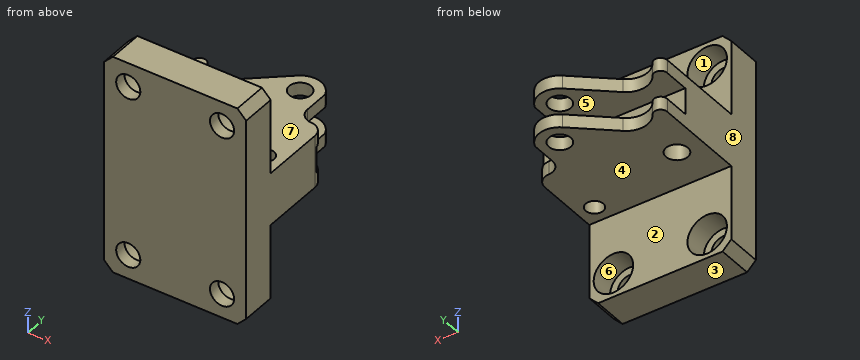
```python
from build123d import *

# Parameters (mm, degrees)
EXTRUDE_1_DEPTH              = 35
SKETCH_2_W                   = 82.468710257
SKETCH_2_H                   = 88.660900106
CUT_EXTRUDE_1_DEPTH          = 40
SKETCH_10_R                  = 2.5
CUT_EXTRUDE_6_DEPTH          = 48.259263975
SKETCH_11_R                  = 2.5
CUT_EXTRUDE_7_DEPTH          = 48.259263975
SKETCH_13_R                  = 2
CUT_EXTRUDE_8_DEPTH          = 48.259263975
FILLET_1_R                   = 3
SKETCH_14_W                  = 32.391015019
SKETCH_14_H                  = 50
EXTRUDE_2_DEPTH              = 8
CHAMFER_1_SIZE               = 2
HOLE_WIZARD_M5_1_D           = 5.5
HOLE_WIZARD_M5_1_CBORE_D     = 9
HOLE_WIZARD_M5_1_CBORE_DEPTH = 5.3


with BuildPart() as part:
    # 草圖1 → 填料-伸長1 (new body)
    with BuildSketch(Plane(origin=(0, 0, 0), x_dir=(0, 0, -1), z_dir=(1, 0, 0))):
        Polygon((-13.9, 3), (-25.9, 3), (-25.9, 38), (-22.9, 38), (-22.9, 18), (-16.9, 18), (-16.9, 38), (-13.9, 38), align=None)
    extrude(amount=-EXTRUDE_1_DEPTH)

    # 草圖2 → 除料-伸長1 (cut)
    with BuildSketch(Plane.XY.offset(13.9)):
        with Locations((-13.573394444, 11.892084287)):
            Rectangle(SKETCH_2_W, SKETCH_2_H)
        with BuildLine():
            Line((-32.391015019, 23.817806702), (-32.391015019, 3))
            Line((-32.391015019, 3), (0, 3))
            Line((0, 3), (0, 20.4))
            Line((0, 20.4), (-2.9, 20.4))
            ThreePointArc((-2.9, 20.4), (-5.021320344, 21.278679656), (-5.9, 23.4))
            Line((-5.9, 23.4), (-5.9, 29.121329309))
            ThreePointArc((-5.9, 29.121329309), (-9.201633351, 32.099001439), (-13.531412968, 31.088891261))
            Line((-13.531412968, 31.088891261), (-22.178800852, 23.645419036))
            ThreePointArc((-22.178800852, 23.645419036), (-26.149318252, 22.485359315), (-29.634828865, 24.712905667))
            ThreePointArc((-29.634828865, 24.712905667), (-31.356390105, 25.322962362), (-32.391015019, 23.817806702))
        make_face(mode=Mode.SUBTRACT)
    extrude(amount=CUT_EXTRUDE_1_DEPTH, mode=Mode.SUBTRACT)

    # 草圖10 → 除料-伸長6 (cut, through all)
    with BuildSketch(Plane.XY.offset(25.9)):
        with Locations((-10.44068936, 27.5)):
            Circle(SKETCH_10_R)
    extrude(amount=-CUT_EXTRUDE_6_DEPTH, mode=Mode.SUBTRACT)

    # 草圖11 → 除料-伸長7 (cut, through all)
    with BuildSketch(Plane.XY.offset(25.9)):
        with Locations((-26.54068936, 12.35)):
            Circle(SKETCH_11_R)
    extrude(amount=-CUT_EXTRUDE_7_DEPTH, mode=Mode.SUBTRACT)

    # 草圖13 → 除料-伸長8 (cut, through all)
    with BuildSketch(Plane.XY.offset(25.9)):
        with Locations((-4, 7)):
            Circle(SKETCH_13_R)
    extrude(amount=-CUT_EXTRUDE_8_DEPTH, mode=Mode.SUBTRACT)

    # 圓角1
    # the kernel refuses this fillet: 3 mm, written as the material it takes off along each edge
    with BuildSketch(Plane(origin=(0, 20.4, 15.402083478), x_dir=(0, -1, 0), z_dir=(0, 0, 1)), Plane(origin=(0, 20.4, 6.402083478), x_dir=(0, -1, 0), z_dir=(0, 0, 1))) as fillet_1_piece_1:
        with BuildLine():
            CenterArc((2.999166609, -3), FILLET_1_R, 90, 89.045026126)
            Line((-0.000416696, -2.95), (-0.300375026, -2.945))
            ThreePointArc((-0.300375026, -2.945), (-0.3, -2.9), (-0.3, 0))
            Line((-0.3, 0), (0, 0.3))
            Line((0, 0.3), (2.999166609, 0.3))
            Line((2.999166609, 0.3), (2.999166609, 0))
        make_face()
    extrude(amount=17.995833044, mode=Mode.SUBTRACT)

    # 草圖14 → 填料-伸長2 (add)
    with BuildSketch(Plane.XZ.offset(-3)):
        with Locations((-16.19550751, 19.9)):
            Rectangle(SKETCH_14_W, SKETCH_14_H)
    extrude(amount=EXTRUDE_2_DEPTH)

    # 導角1
    chamfer_1_edges = [part.edges().sort_by_distance(p)[0] for p in [
        (-32.391015019, -1, -5.1),
        (0, -1, -5.1),
        (-32.391015019, -1, 44.9),
        (0, -1, 44.9),
    ]]
    chamfer(chamfer_1_edges, length=CHAMFER_1_SIZE)

    # M5 內六角圓柱頭螺釘的柱孔1 (through all)
    with Locations(Plane(origin=(0, 3, 0), x_dir=(1, 0, 0), z_dir=(0, 1, 0))):
        with Locations((-26.891015019, -0.4), (-5.5, -0.4), (-5.5, -39.4), (-26.891015019, -39.4)):
            CounterBoreHole(HOLE_WIZARD_M5_1_D / 2, HOLE_WIZARD_M5_1_CBORE_D / 2, HOLE_WIZARD_M5_1_CBORE_DEPTH)


solid = part.part
```
CAD build for the part. Positions are in the model's coordinates, mm. Face numbers are marked on the shaded views. A direction names the side the tool comes from. Round coordinates to 2 decimals unless told otherwise and drop trailing zeros. Order: outer loops, then holes, each group sorted by start corner. A loop starts at its lowest first (then second) coordinate and runs counter-clockwise, first axis right, second up.
Q1. Which spindle directions (+Z, -Z, +X, -X, +Y, -Y) get a long thin tool onto all of the face, cutting with end or side? Do the marked faces 4, 5, 6, 7 and 8. Say none if no direction does.
Q2. Slice it at A-A (z = 39.4). Write the cut outline in (x, y), and give its area (3 significant figures).
Q3. Wall check: L1, parallel to Z at x = -5.5, y = -4.1; L2, parallel to Z at x = -6.5, y = 23.5; L3, parallel to X at y = -0.5, z = 35.5 (3 decimals). Give the ranges that are in metal, low to high.
Q4. Slice it at B-B (y = 12.35). Write the cut outline in (x, z).
Q5. Slice it at D-D (y = 27.5). Write the cut outline in (x, z).
Q6. Slice it at C-C (x = -25). State how many separate pieces and enclosed holes the cut face has, and give its area (3 significant figures).
Q7. Drop flat-ended pins along their axis: pin 1 (6 mm diameter, centred on y = 4, z = 39, fed in from -X); pin 2 (0.9 mm diameter, centred on y = 27, z = 24.5, fed in from +X); pin 3 (11.5 mm diameter, centred on x = -26.89, z = 0.4, fed in from +Y); pin 4 (10 mm diameter, centred on x = -24.5, y = 5, fed in from +Z). Give the stop position or say it passes through.
Q8. Two-plate mould, pull along Z, no slides. Class the marked faces 1, 2 and 3: pulls with the +Z half, pulls with the -Z half, needs draft (parallel to the pull), parting line crosses it, or undercut.
Results below:
1. face 4: -Z, +X, -X, +Y
1. face 5: +X, -X, +Y
1. face 6: +Y
1. face 7: +Z, +X, -X, +Y
1. face 8: +Z, -Z, -X, +Y, -Y
2. outline: (-32.39, -5) - (-29.64, -5) - (-29.64, -2.3) - (-31.39, -2.3) - (-31.39, 3) - (-32.39, 3) - close; (-24.14, -5) - (-8.25, -5) - (-8.25, -2.3) - (-10, -2.3) - (-10, 3) - (-22.39, 3) - (-22.39, -2.3) - (-24.14, -2.3) - close; (-2.75, -5) - (0, -5) - (0, 3) - (-1, 3) - (-1, -2.3) - (-2.75, -2.3) - close
2. area: 134 mm2
3. L1: z = -5.1 to -2.35, 3.15 to 36.65, 42.15 to 44.9
3. L2: z = 13.9 to 16.9, 22.9 to 25.9
3. L3: x = -32.391 to -29.136, -24.646 to -7.745, -3.255 to 0
4. outline: (-32.39, 13.9) - (-29.04, 13.9) - (-29.04, 25.9) - (-32.39, 25.9) - close; (-24.04, 13.9) - (0, 13.9) - (0, 25.9) - (-24.04, 25.9) - close
5. outline: (-17.7, 13.9) - (-12.94, 13.9) - (-12.94, 16.9) - (-17.7, 16.9) - close; (-17.7, 22.9) - (-12.94, 22.9) - (-12.94, 25.9) - (-17.7, 25.9) - close; (-7.94, 13.9) - (-5.9, 13.9) - (-5.9, 16.9) - (-7.94, 16.9) - close; (-7.94, 22.9) - (-5.9, 22.9) - (-5.9, 25.9) - (-7.94, 25.9) - close
6. separate pieces: 4
6. enclosed holes: 0
6. area: 451 mm2
7. pin 1: stops at x = -32.39
7. pin 2: stops at x = -5.9
7. pin 3: stops at y = 3
7. pin 4: stops at z = 44.9
8. face 1: undercut
8. face 2: needs draft
8. face 3: pulls with the -Z half
